```python
from build123d import *

# Parameters (mm, degrees)
SKETCH1_W                         = 32.4
SKETCH1_H                         = 30
SKETCH1_R                         = 1.75
BOSS_EXTRUDE1_DEPTH               = 25
SKETCH2_R                         = 4
CUT_EXTRUDE1_DEPTH                = 20
SKETCH3_W                         = 32.4
SKETCH3_H                         = 30
SKETCH3_R                         = 4
BOSS_EXTRUDE2_DEPTH               = 3
SKETCH4_W                         = 32.4
SKETCH4_H                         = 30
BOSS_EXTRUDE3_DEPTH               = 23.5
SKETCH5_R                         = 1.25
CUT_EXTRUDE2_DEPTH                = 2.45
SKETCH6_W                         = 22
SKETCH6_H                         = 4
CUT_EXTRUDE3_DEPTH                = 5.15
SKETCH7_W                         = 15
SKETCH7_H                         = 10
BOSS_EXTRUDE4_DEPTH               = 10
SKETCH8_W                         = 5.6
SKETCH8_H                         = 10
CUT_EXTRUDE4_DEPTH                = 15
CHAMFER1_SIZE                     = 1
SKETCH11_R                        = 1
CUT_EXTRUDE5_DEPTH                = 5
CHAMFER3_SIZE                     = 1
BOSS_EXTRUDE6_DEPTH               = 15
CHAMFER5_SIZE                     = 1
F_3_32_0_140625_DOWEL_HOLE1_D     = 3.571875
F_3_32_0_140625_DOWEL_HOLE1_DEPTH = 12.7
F_3_32_0_140625_DOWEL_HOLE1_TIP   = 1.073099512
SKETCH19_W                        = 5
SKETCH19_H                        = 7
BOSS_EXTRUDE7_DEPTH               = 25


with BuildPart() as part:
    # Sketch1 → Boss-Extrude1 (new body)
    with BuildSketch(Plane(origin=(0, 0, 0), x_dir=(1, 0, 0), z_dir=(0, 1, 0))):
        with Locations((16.2, -15)):
            Rectangle(SKETCH1_W, SKETCH1_H)
        with Locations((6.2, -5)):
            Circle(SKETCH1_R, mode=Mode.SUBTRACT)
        with Locations((26.2, -5)):
            Circle(SKETCH1_R, mode=Mode.SUBTRACT)
        with Locations((26.2, -25)):
            Circle(SKETCH1_R, mode=Mode.SUBTRACT)
        with Locations((6.2, -25)):
            Circle(SKETCH1_R, mode=Mode.SUBTRACT)
    extrude(amount=BOSS_EXTRUDE1_DEPTH)

    # Sketch2 → Cut-Extrude1 (cut)
    with BuildSketch(Plane(origin=(0, 25, 0), x_dir=(1, 0, 0), z_dir=(0, 1, 0))):
        with Locations((16.2, -15)):
            Circle(SKETCH2_R)
    extrude(amount=-CUT_EXTRUDE1_DEPTH, mode=Mode.SUBTRACT)

    # Sketch3 → Boss-Extrude2 (add)
    with BuildSketch(Plane(origin=(0, 25, 0), x_dir=(1, 0, 0), z_dir=(0, 1, 0))):
        with Locations((16.2, -15)):
            Rectangle(SKETCH3_W, SKETCH3_H)
        Polygon((3, -20), (3, -10), (3, -2), (11, -2), (21.4, -2), (29.4, -2), (29.4, -10), (29.4, -20), (29.4, -28), (21.4, -28), (11, -28), (3, -28), align=None, mode=Mode.SUBTRACT)
        with BuildLine():
            ThreePointArc((11, -2), (8.656854249, -7.656854249), (3, -10))
            Line((3, -10), (3, -20))
            ThreePointArc((3, -20), (8.656854249, -22.343145751), (11, -28))
            Line((11, -28), (21.4, -28))
            ThreePointArc((21.4, -28), (23.743145751, -22.343145751), (29.4, -20))
            Line((29.4, -20), (29.4, -10))
            ThreePointArc((29.4, -10), (23.743145751, -7.656854249), (21.4, -2))
            Line((21.4, -2), (11, -2))
        make_face()
        with Locations((16.2, -15)):
            Circle(SKETCH3_R, mode=Mode.SUBTRACT)
    extrude(amount=BOSS_EXTRUDE2_DEPTH)

    # Sketch4 → Boss-Extrude3 (add)
    with BuildSketch(Plane(origin=(0, 28, 0), x_dir=(1, 0, 0), z_dir=(0, 1, 0))):
        with Locations((16.2, -15)):
            Rectangle(SKETCH4_W, SKETCH4_H)
        with BuildLine():
            Line((5.15, -20.294320277), (5.15, -9.705679723))
            ThreePointArc((5.15, -9.705679723), (4.085025855, -9.926078406), (3, -10))
            Line((3, -10), (3, -2))
            Line((3, -2), (11, -2))
            ThreePointArc((11, -2), (10.996832804, -2.225089113), (10.987333723, -2.45))
            Line((10.987333723, -2.45), (21.412666277, -2.45))
            ThreePointArc((21.412666277, -2.45), (21.403167196, -2.225089113), (21.4, -2))
            Line((21.4, -2), (29.4, -2))
            Line((29.4, -2), (29.4, -10))
            ThreePointArc((29.4, -10), (28.314974145, -9.926078406), (27.25, -9.705679723))
            Line((27.25, -9.705679723), (27.25, -20.294320277))
            ThreePointArc((27.25, -20.294320277), (28.314974145, -20.073921594), (29.4, -20))
            Line((29.4, -20), (29.4, -28))
            Line((29.4, -28), (21.4, -28))
            ThreePointArc((21.4, -28), (21.403167196, -27.774910887), (21.412666277, -27.55))
            Line((21.412666277, -27.55), (10.987333723, -27.55))
            ThreePointArc((10.987333723, -27.55), (10.996832804, -27.774910887), (11, -28))
            Line((11, -28), (3, -28))
            Line((3, -28), (3, -20))
            ThreePointArc((3, -20), (4.085025855, -20.073921594), (5.15, -20.294320277))
        make_face(mode=Mode.SUBTRACT)
    extrude(amount=BOSS_EXTRUDE3_DEPTH)

    # Sketch5 → Cut-Extrude2 (cut)
    with BuildSketch(Plane(origin=(0, 0, 0), x_dir=(-1, 0, 0), z_dir=(0, 0, -1))):
        with Locations((-22.2, 49)):
            Circle(SKETCH5_R)
        with Locations((-10.2, 34)):
            Circle(SKETCH5_R)
    extrude(amount=-CUT_EXTRUDE2_DEPTH, mode=Mode.SUBTRACT)

    # Sketch6 → Cut-Extrude3 (cut)
    with BuildSketch(Plane.ZY):
        with Locations((15, 30)):
            Rectangle(SKETCH6_W, SKETCH6_H)
    extrude(amount=-CUT_EXTRUDE3_DEPTH, mode=Mode.SUBTRACT)

    # Sketch7 → Boss-Extrude4 (add)
    with BuildSketch(Plane(origin=(32.4, 0, 0), x_dir=(0, 0, -1), z_dir=(1, 0, 0))):
        with Locations((-15, 46.5)):
            Rectangle(SKETCH7_W, SKETCH7_H)
    extrude(amount=BOSS_EXTRUDE4_DEPTH)

    # Sketch8 → Cut-Extrude4 (cut)
    with BuildSketch(Plane(origin=(0, 51.5, 0), x_dir=(1, 0, 0), z_dir=(0, 1, 0))):
        with Locations((37.4, -15)):
            Rectangle(SKETCH8_W, SKETCH8_H)
    extrude(amount=-CUT_EXTRUDE4_DEPTH, mode=Mode.SUBTRACT)

    # Chamfer1
    chamfer1_edges = [part.edges().sort_by_distance(p)[0] for p in [
        (34.6, 46.5, 20),
        (40.2, 46.5, 20),
    ]]
    chamfer(chamfer1_edges, length=CHAMFER1_SIZE)

    # Sketch11 → Cut-Extrude5 (cut)
    with BuildSketch(Plane.XY.offset(30)):
        with Locations((7.535754107, 46.7)):
            Circle(SKETCH11_R)
        with Locations((25.535754107, 46.7)):
            Circle(SKETCH11_R)
        with Locations((7.535754107, 36.7)):
            Circle(SKETCH11_R)
        with Locations((25.535754107, 36.7)):
            Circle(SKETCH11_R)
        with Locations((16.535754107, 41.7)):
            Circle(SKETCH11_R)
    extrude(amount=-CUT_EXTRUDE5_DEPTH, mode=Mode.SUBTRACT)

    # Chamfer3
    chamfer3_edges = [part.edges().sort_by_distance(p)[0] for p in [
        (32.4, 46.5, 7.5),
        (32.4, 46.5, 22.5),
        (32.4, 41.5, 15),
        (42.4, 46.5, 7.5),
        (42.4, 46.5, 22.5),
    ]]
    chamfer(chamfer3_edges, length=CHAMFER3_SIZE)

    # Sketch15 → Boss-Extrude6 (add)
    with BuildSketch(Plane(origin=(0, 51.5, 0), x_dir=(1, 0, 0), z_dir=(0, 1, 0))):
        Polygon((32.4, -7.5), (41.4, -7.5), (42.4, -8.5), (42.4, -21.5), (41.4, -22.5), (32.4, -22.5), align=None)
        Polygon((34.6, -10), (34.6, -19), (35.6, -20), (39.2, -20), (40.2, -19), (40.2, -10), align=None, mode=Mode.SUBTRACT)
    extrude(amount=BOSS_EXTRUDE6_DEPTH)

    # Chamfer5
    chamfer5_edges = [part.edges().sort_by_distance(p)[0] for p in [
        (32.4, 59, 7.5),
        (32.4, 59, 22.5),
    ]]
    chamfer(chamfer5_edges, length=CHAMFER5_SIZE)

    # 3/32 (0.140625) Dowel Hole1
    with Locations(Plane.XY.offset(30)):
        with Locations((5.645879952, 25.599824203), (15.645879952, 3.599824203)):
            Hole(F_3_32_0_140625_DOWEL_HOLE1_D / 2, depth=F_3_32_0_140625_DOWEL_HOLE1_DEPTH)
            with Locations((0, 0, -(F_3_32_0_140625_DOWEL_HOLE1_DEPTH + F_3_32_0_140625_DOWEL_HOLE1_TIP / 2))):  # 118° drill point
                Cone(0, F_3_32_0_140625_DOWEL_HOLE1_D / 2, F_3_32_0_140625_DOWEL_HOLE1_TIP, mode=Mode.SUBTRACT)

    # Sketch19 → Boss-Extrude7 (add)
    with BuildSketch(Plane(origin=(0, 0, 0), x_dir=(-1, 0, 0), z_dir=(0, 0, -1))):
        with Locations((-2.83125, 32.5777)):
            Rectangle(SKETCH19_W, SKETCH19_H)
    extrude(amount=BOSS_EXTRUDE7_DEPTH)


solid = part.part
```
Check sheet for the modelled part. Datum: model origin and axes. Units: mm. A direction names the side the tool comes from. Coordinates: 2 decimals unless noted, no trailing zeros. Write each loop counter-clockwise with the first axis right and the second up, starting at its lowest first coordinate (ties: lowest second). Pieces come first, ordered by that corner, then holes. Notation, with made-up numbers: (-6, 26.5) -> (-1, 26.5) arc R18 ccw to (-1, 60.5) -> close; hole circle Ø8 at (-8, -36). An arc over 180 degrees is marked (long way). Use a Markdown table: item, result.
1. Go/stop test with flat-tipped pins: pin 1 Ø2 at (x, z) = (27.5, 18.5) entering from +Y; pin 2 Ø3 at (x, y) = (35.5, 58.5) entering from +Z; pin 3 Ø4 at (x, z) = (8, 8.5) entering from +Y; pin 4 Ø10 at (y, z) = (59, 2) entering from -X. Record where each tip stops, or that it passes through.
Reported:
| item | result |
|---|---|
| pin 1 | stops at y = 51.5 |
| pin 2 | stops at z = 22.5 |
| pin 3 | stops at y = 28 |
| pin 4 | passes through |
2. Release check for a two-part mould opening along Y. For faces 4 (the flat face through (3, 36.078, -12)), 5 (the cylindrical face through (7.319, 35.724, 29.014)), 6 (the cylindrical face through (5.972, 12.325, 23.265)), 7 (the flat face through (13, 28, 12)) record: pulls with the +Y half, pulls with the -Y half, needs draft (parallel to the pull), parting line crosses it, or undercut.
Reported:
| item | result |
|---|---|
| face 4 | pulls with the +Y half |
| face 5 | undercut |
| face 6 | needs draft |
| face 7 | undercut |
3. Sectioned sample at D-D (y = 55). Enter the section's corners in (x, z).
Reported:
| item | result |
|---|---|
| outline | (32.4, 8.5) -> (33.4, 7.5) -> (41.4, 7.5) -> (42.4, 8.5) -> (42.4, 21.5) -> (41.4, 22.5) -> (33.4, 22.5) -> (32.4, 21.5) -> close; hole (34.6, 10) -> (40.2, 10) -> (40.2, 19) -> (39.2, 20) -> (35.6, 20) -> (34.6, 19) -> close |
4. Sectioned sample at B-B (y = 16). Enter the section's corners in (x, z), plus the area to 3 significant figures.
Reported:
| item | result |
|---|---|
| outline | (0, 0) -> (32.4, 0) -> (32.4, 30) -> (0, 30) -> close; hole circle Ø3.5 at (6.2, 5); hole circle Ø3.5 at (6.2, 25); hole circle Ø8 at (16.2, 15); hole circle Ø3.5 at (26.2, 5); hole circle Ø3.5 at (26.2, 25) |
| area | 883 mm2 |
5. Sectioned sample at C-C (z = 15). Enter the section's corners in (x, y).
Reported:
| item | result |
|---|---|
| outline | (0, 0) -> (32.4, 0) -> (32.4, 40.5) -> (33.4, 41.5) -> (34.6, 41.5) -> (34.6, 66.5) -> (32.4, 66.5) -> (32.4, 51.5) -> (27.25, 51.5) -> (27.25, 28) -> (20.2, 28) -> (20.2, 5) -> (12.2, 5) -> (12.2, 28) -> (0, 28) -> close; (0, 32) -> (5.15, 32) -> (5.15, 51.5) -> (0, 51.5) -> close; (40.2, 41.5) -> (42.4, 41.5) -> (42.4, 66.5) -> (40.2, 66.5) -> close |
6. Scan lines: line 1 along Z through (x, y) = (6.2, 6.25); line 2 along X through (y, z) = (49.5, 15); line 3 along Z through (x, y) = (37, 44). Record each from-to range of solid material in increasing order.
Reported:
| item | result |
|---|---|
| line 1 | z = 0 to 3.25, 6.75 to 23.25, 26.75 to 30 |
| line 2 | x = 0 to 5.15, 27.25 to 34.6, 40.2 to 42.4 |
| line 3 | z = 7.5 to 10, 20 to 22.5 |
7. Tool access check on faces 1 (the flat face through (5.15, 42, 15)), 2 (the flat face through (3, 29.078, -12)), 3 (the cylindrical face through (16.997, 40.813, 28.792)). Record the directions out of +Z, -Z, +X, -X, +Y, -Y that give a thin tool (end or side, any length) a straight path to the whole face; none if there is none.
Reported:
| item | result |
|---|---|
| face 1 | +Y |
| face 2 | -Z, +X, -X, -Y |
| face 3 | +Z |
8. Sectioned sample at A-A (z = 25). Enter the section's corners in (x, y).
Reported:
| item | result |
|---|---|
| outline | (0, 0) -> (4.45, 0) -> (4.45, 24.27) arc R1.79 cw to (3.96, 25) -> (3, 25) -> (3, 28) -> (0, 28) -> close; (0, 32) -> (3, 32) -> (3, 51.5) -> (0, 51.5) -> close; (7.95, 0) -> (24.45, 0) -> (24.45, 25) -> (21.98, 25) -> (21.98, 28) -> (10.42, 28) -> (10.42, 25) -> (7.95, 25) -> close; (27.95, 0) -> (32.4, 0) -> (32.4, 51.5) -> (29.4, 51.5) -> (29.4, 25) -> (27.95, 25) -> close; hole circle Ø3.57 at (15.65, 3.6) |
